Autodesk Fusion 360 part; units mm, degrees
sketch "Sketch2" plane through (0, 0, 0) normal (0, 1, 0) x (1, 0, 0)
  line L0 (730, 360) -> (-730, 360)
  line L1 (-730, 360) -> (-730, -360)
  line L2 (-730, -360) -> (730, -360)
  line L3 (730, -360) -> (730, 360)
  line L4 (730, 360) -> (-730, -360) construction
  line L5 (-730, 360) -> (730, -360) construction
  line L6 (-730, -360) -> (-10, -360)
  line L7 (-10, -360) -> (-10, 140)
  line L8 (-10, 140) -> (-730, 140)
  line L9 (-730, 140) -> (-730, -360)
  line L10 (230, 2.3053) -> (230, 122.3053)
  line L11 (230, 122.3053) -> (730, 122.3053)
  line L12 (230, -117.6947) -> (730, -117.6947)
  arc A0 (245.8705, 121.2512) -> (238.1032, -117.4208) centre (230, 2.3053) ccw
  dimension "d7" = 1460
  dimension "d8" = 720
  dimension "d9" = 720
  dimension "d10" = 500
  dimension "d11" = 240
  dimension "d12" = 500
  dimension "d13" = 90
extrude "Extrude1" add sketch "Sketch2" along normal blind 250 contours L0 L1 L2 L3 L7 L8 L11 L12 A0 | L1 L2 L6 L7 L8 L9
extrude "Extrude2" cut sketch "Sketch2" along normal blind 60 contours L1 L2 L6 L7 L8 L9
sketch "Sketch3" plane through (0, 250, 0) normal (0, 1, 0) x (-1, 0, 0)
  arc A0 (-230, -122.3053) -> (-230, 117.6947) centre (-230, -2.3053) ccw
  line L0 (-230, -122.3053) -> (-730, -122.3053)
  line L1 (-730, -122.3053) -> (-730, -360)
  line L2 (-730, -360) -> (730, -360)
  line L3 (730, -360) -> (730, 360)
  line L4 (730, 360) -> (-730, 360)
  line L5 (-730, 360) -> (-730, 117.6947)
  line L6 (-730, 117.6947) -> (-230, 117.6947)
  line L7 (730, 360) -> (370, 360)
  line L8 (370, 360) -> (370, -360)
  line L9 (370, -360) -> (730, -360)
  line L10 (730, -360) -> (730, 360)
  dimension "d18" = 360
extrude "Extrude3" add sketch "Sketch3" along normal blind 650 contours L2 L3 L4 L7 L8 L9 L10
sketch "Sketch4" plane through (-730, 0, 0) normal (-1, 0, 0) x (0, 0, 1)
  line L0 (-140, 0) -> (-140, 60)
  line L1 (-140, 60) -> (360, 60)
  line L2 (360, 60) -> (360, 900)
  line L3 (360, 900) -> (-360, 900)
  line L4 (-360, 900) -> (-360, 0)
  line L5 (-360, 0) -> (-140, 0)
  circle A0 centre (0, 480) radius 120
  circle A1 centre (0, 480) radius 300
  line L6 (-360, 900) -> (360, 900)
  line L7 (360, 900) -> (360, 660)
  line L8 (360, 660) -> (-360, 660)
  line L9 (-360, 660) -> (-360, 900)
  line L10 (360, 60) -> (-360, 60)
  line L11 (-360, 60) -> (-360, 300)
  line L12 (-360, 300) -> (360, 300)
  line L13 (360, 300) -> (360, 60)
  dimension "d21" = 240
  dimension "d22" = 600
  dimension "d23" = 480
  dimension "d24" = 240
  dimension "d25" = 240
extrude "Extrude4" cut sketch "Sketch4" against normal through all contours A0
extrude "Extrude5" cut sketch "Sketch4" against normal blind 120 contours L2 A1 L8 L12 | L4 A1 L8 L12 | A1 L8 L12 | A1 L12 | A1 L8
Check sheet for the modelled part. Datum: model origin and axes. Units: mm. A direction names the side the tool comes from. Round coordinates to 2 decimals unless told otherwise and drop trailing zeros. Loops run counter-clockwise (first coordinate to the right, second up) from the corner with the lowest first, then second, coordinate; pieces in that order, holes last. Notation, with made-up numbers: (27, -16) -> (74, -16) arc R6 ccw to (74, -10) -> close; hole circle Ø2 at (13, 38.25). An arc over 180 degrees is marked (long way). Answer in a Markdown table with one row per item.
Q1. Sectioned sample at B-B on y = 480. Enter the section's corners in (x, z), then the cut area to 3 significant figures.
Data:
| item | result |
|---|---|
| outline | (-610, -360) -> (-370, -360) -> (-370, -120) -> (-610, -120) -> close; (-610, 120) -> (-370, 120) -> (-370, 360) -> (-610, 360) -> close |
| area | 115,000 mm^2 |
Q2. Sectioned sample at D-D on z = 306.5. Enter the section's corners in (x, y), then the cut area to 3 significant figures.
Data:
| item | result |
|---|---|
| outline | (-730, 60) -> (-10, 60) -> (-10, 0) -> (730, 0) -> (730, 250) -> (-370, 250) -> (-370, 900) -> (-730, 900) -> (-730, 660) -> (-610, 660) -> (-610, 300) -> (-730, 300) -> close |
| area | 513,000 mm^2 |
Q3. Release check for a two-part mould opening along Y. For faces 1 (the face through (-730, 805, -5)), 2 (the face through (50, 250, -5)), 3 (the face through (152, 0, -165)), 4 (the face through (-671, 660, -299)) record: released by +Y, released by -Y, zero draft, split by the parting line, or undercut.
Data:
| item | result |
|---|---|
| face 1 | zero draft |
| face 2 | released by +Y |
| face 3 | released by -Y |
| face 4 | undercut |
Q4. Set-up check for faces 5 (the face through (-370, 643, 5)), 6 (the face through (-671, 300, 299)), 7 (the face through (476, 123, -122.305)), 8 (the face through (-375, 60, 106)), 9 (the face through (-670.84, 180.025, -3.895)): record each of +Z, -Z, +X, -X, +Y, -Y from which the full face is reachable in a straight line by a thin tool's end or side.
Data:
| item | result |
|---|---|
| face 5 | +Z, -Z, +X, +Y |
| face 6 | +Z, -Z, -X |
| face 7 | +X, +Y, -Y |
| face 8 | +Z, -X, -Y |
| face 9 | -X |
Q5. Sectioned sample at A-A on x = 410.5. Enter the section's corners in (y, z), then the cut area to 3 significant figures.
Data:
| item | result |
|---|---|
| outline | (0, -360) -> (250, -360) -> (250, -122.31) -> (0, -122.31) -> close; (0, 117.69) -> (250, 117.69) -> (250, 360) -> (0, 360) -> close |
| area | 120,000 mm^2 |
Q6. Thickness scan on L1, parallel to Y at x = -497, z = 0; L2, parallel to Z at x = 502, y = 187; L3, parallel to X at y = 782, z = 280. Record the ranges inside material, lowest first.
Data:
| item | result |
|---|---|
| L1 | y = 60 to 360, 600 to 900 |
| L2 | z = -360 to -122.31, 117.69 to 360 |
| L3 | x = -730 to -370 |
Q7. Sectioned sample at C-C on x = -587.5. Enter the section's corners in (y, z), then the cut area to 3 significant figures.
Data:
| item | result |
|---|---|
| outline | (0, -360) -> (900, -360) -> (900, 360) -> (60, 360) -> (60, -140) -> (0, -140) -> close; hole circle Ø240 at (480, 0) |
| area | 573,000 mm^2 |
Q8. Go/stop test with flat-tipped pins: P1, Ø10, axis at y = 145, z = -86, coming from the +X side; P2, Ø1, axis at y = 688.5, z = -92.5, coming from the -X side; P3, Ø12, axis at x = -230.5, z = -66.5, coming from the -Y side. Record where each tip stops, or that it passes through.
Data:
| item | result |
|---|---|
| P1 | stops at x = 149.17 |
| P2 | stops at x = -610 |
| P3 | stops at y = 60 |
